Part model, mm, in its own coordinate system. A direction names the side the tool comes from. Coordinates: 2 decimals unless noted, no trailing zeros. Write each loop counter-clockwise with the first axis right and the second up, starting at its lowest first coordinate (ties: lowest second). Pieces come first, ordered by that corner, then holes. Notation, with made-up numbers: (-9, 55.25) -> (37, 55.25) arc R35 ccw to (37, 94.25) -> close; hole circle Ø10 at (-11.75, -12.5). An arc over 180 degrees is marked (long way). Write item = value, one per line. Start each with the question number.
Q1. Tool access for faces 1 (the flat face through (-22, 15, 37)), 2 (the flat face through (46.4, 5, 19.2)): list every direction of +Z, -Z, +X, -X, +Y, -Y with a clear straight run to the whole face (end or side of a thin tool).
Q2. Band-saw the part on B-B, the plane x = 0. List the corners of the cut face in (y, z).
Q3. Probe line 1 (Z direction, x = 0, y = 5.5); line 2 (Z direction, x = 0, y = 1.3). List the from-to ranges inside material, lowest first.
Q4. Pin check, flat tips, straight feed: P1, Ø3, axis at x = -39, y = 5, coming from the +Z side; P2, Ø2, axis at y = 7.5, z = -18.5, coming from the +X side; P3, Ø6, axis at y = 8.5, z = -5, coming from the +X side. Stop position of each tip, or through.
Q5. Band-saw the part on C-C, the plane y = 7.5. List the corners of the cut face in (x, z).
Q6. Band-saw the part on D-D, the plane z = -45. List the corners of the cut face in (x, y), plus the area to 3 significant figures.
Q7. Band-saw the part on A-A, the plane z = 0. List the corners of the cut face in (x, y), plus the area to 3 significant figures.
from build123d import *

# Parameters (mm, degrees)
SKETCH1_R           = 52.5
BOSS_EXTRUDE1_DEPTH = 5
SKETCH2_R           = 50
SKETCH2_R_2         = 42.5
BOSS_EXTRUDE2_DEPTH = 10
SKETCH3_R           = 42.5
CUT_EXTRUDE1_DEPTH  = 6


with BuildPart() as part:
    # Sketch1 → Boss-Extrude1 (new body)
    with BuildSketch(Plane(origin=(0, 0, 0), x_dir=(1, 0, 0), z_dir=(0, 1, 0))):
        Circle(SKETCH1_R)
    extrude(amount=BOSS_EXTRUDE1_DEPTH)

    # Sketch2 → Boss-Extrude2 (add)
    with BuildSketch(Plane(origin=(0, 5, 0), x_dir=(1, 0, 0), z_dir=(0, 1, 0))):
        Circle(SKETCH2_R)
        Circle(SKETCH2_R_2, mode=Mode.SUBTRACT)
    extrude(amount=BOSS_EXTRUDE2_DEPTH)

    # Sketch3 → Cut-Extrude1 (cut, through all)
    with BuildSketch(Plane(origin=(0, 5, 0), x_dir=(1, 0, 0), z_dir=(0, 1, 0))):
        Circle(SKETCH3_R)
    extrude(amount=-CUT_EXTRUDE1_DEPTH, mode=Mode.SUBTRACT)


solid = part.part
Ans:
q1.face_1 = +Z, -Z, +X, -X, +Y
q1.face_2 = +Y
q2.outline = (0, -52.5) -> (5, -52.5) -> (5, -50) -> (15, -50) -> (15, -42.5) -> (0, -42.5) -> close; (0, 42.5) -> (15, 42.5) -> (15, 50) -> (5, 50) -> (5, 52.5) -> (0, 52.5) -> close
q3.line_1 = -50 to -42.5, 42.5 to 50
q3.line_2 = -52.5 to -42.5, 42.5 to 52.5
q4.P1 = 36.74
q4.P2 = 46.84
q4.P3 = 49.96
q5.outline = circle Ø100 at (0, 0); hole circle Ø85 at (0, 0)
q6.outline = (-27.04, 0) -> (27.04, 0) -> (27.04, 5) -> (21.79, 5) -> (21.79, 15) -> (-21.79, 15) -> (-21.79, 5) -> (-27.04, 5) -> close
q6.area = 706 mm2
q7.outline = (-52.5, 0) -> (-42.5, 0) -> (-42.5, 15) -> (-50, 15) -> (-50, 5) -> (-52.5, 5) -> close; (42.5, 0) -> (52.5, 0) -> (52.5, 5) -> (50, 5) -> (50, 15) -> (42.5, 15) -> close
q7.area = 250 mm2
